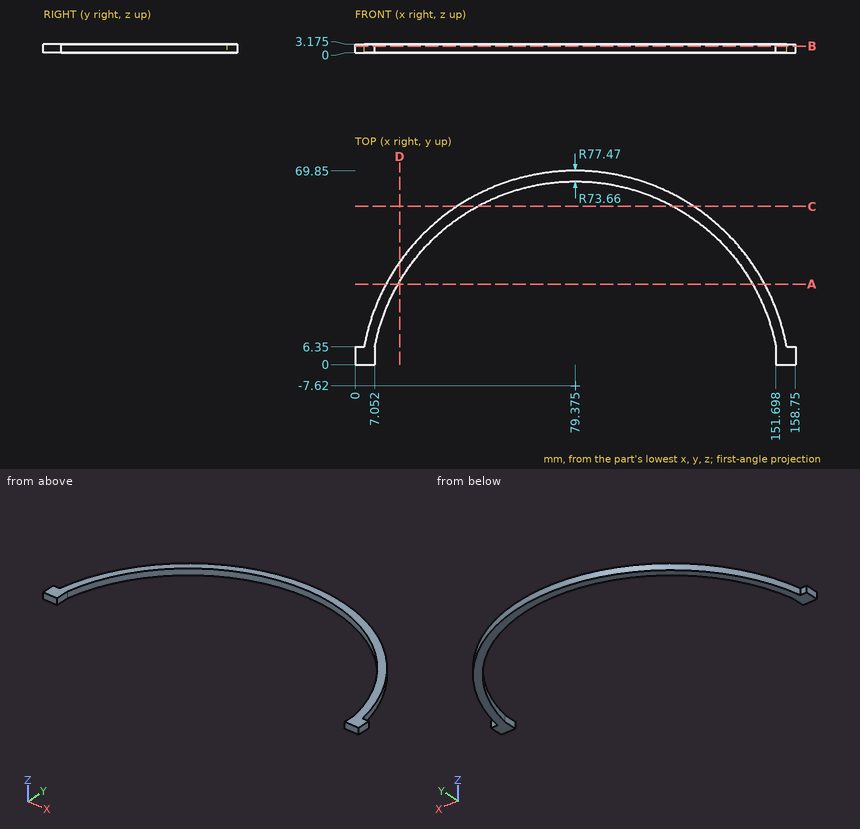
Answer from the drawing. Dimensions are ordinates in mm from the lowest x, y and z of the part. Round coordinates to 2 decimals unless told otherwise and drop trailing zeros. Loops run counter-clockwise (first coordinate to the right, second up) from the corner with the lowest first, then second, coordinate; pieces in that order, holes last.
Q1. Section B-B on z = 2.45 is taken. Write down the section's boundary in (x, y) (3 decimals), and give its area (3 significant figures).
Q2. Section C-C on y = 57 is taken. Write down the section's boundary in (x, z) (3 decimals), and give its area (3 significant figures).
Q3. Section A-A on y = 29 is taken. Write down the section's boundary in (x, z) (1 decimal), and give its area (3 significant figures).
Q4. Consider probe 1 along X at (y, z) = (5, 0.45); probe 2 along X at (y, z) = (53, 3); probe 3 along Y at (x, z) = (99.5, 2.65). Determine where each line is inside the solid, lowest interval first.
Q5. Section D-D on x = 16 is taken. Write down the section's boundary in (y, z) (1 decimal).
Q6. Each of these flat-tipped pins is pushed along its axis until it touches: pin 1 (1.6 mm diameter, centred on x = 156.5, z = 1, fed in from +Y); pin 2 (1.5 mm diameter, centred on x = 79.5, z = 3, fed in from -Y); pin 3 (1 mm diameter, centred on y = 11, z = 1.5, fed in from -X). Where does it stop, or does it pass through?
Output:
1. outline: (0, 0) - (7.052, 0) - (7.052, 6.35) arc R73.66 cw to (151.698, 6.35) - (151.698, 0) - (158.75, 0) - (158.75, 6.35) - (155.575, 6.35) arc R77.47 ccw to (3.175, 6.35) - (0, 6.35) - close
1. area: 887 mm2
2. outline: (36.645, 0) - (44.019, 0) - (44.019, 3.175) - (36.645, 3.175) - close; (114.731, 0) - (122.105, 0) - (122.105, 3.175) - (114.731, 3.175) - close
2. area: 46.8 mm2
3. outline: (11.1, 0) - (15.5, 0) - (15.5, 3.2) - (11.1, 3.2) - close; (143.3, 0) - (147.6, 0) - (147.6, 3.2) - (143.3, 3.2) - close
3. area: 27.7 mm2
4. probe 1: x = 0 to 7.05, 151.7 to 158.75
4. probe 2: x = 31.14 to 37.53, 121.22 to 127.61
4. probe 3: y = 63.24 to 67.19
5. outline: (29.9, 0) - (36.9, 0) - (36.9, 3.2) - (29.9, 3.2) - close
6. pin 1: stops at y = 6.35
6. pin 2: stops at y = 66.03
6. pin 3: stops at x = 4.05
